Drawing for the job (mm, zero at the part's lowest x, y, z). A direction names the side the tool comes from. Round coordinates to 2 decimals unless told otherwise and drop trailing zeros. Order: outer loops, then holes, each group sorted by start corner. A loop starts at its lowest first (then second) coordinate and runs counter-clockwise, first axis right, second up. Notation, with made-up numbers: (-0.75, 88.25) -> (21.25, 88.25) arc R20 cw to (21.25, 97.25) -> close; hole circle Ø4 at (-38.75, 22.25). An arc over 180 degrees is marked (long way). Use CSV: the item, a comma, the result in double quotes.
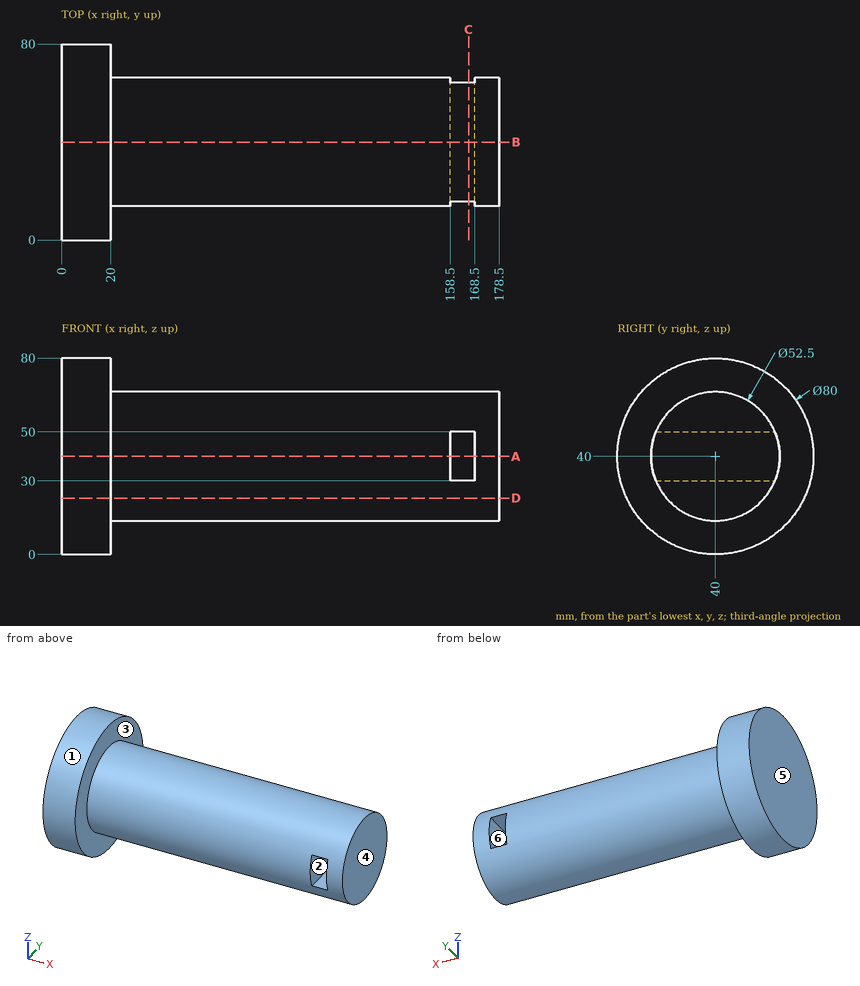
Q1. Cut at C-C (x = 166). Give the cut face in (y, z).
From the geometry:
outline,"(15.73, 30) arc R26.25 ccw to (64.27, 30) -> close; (15.73, 50) -> (64.27, 50) arc R26.25 ccw to start"
Q2. Which spindle directions (+Z, -Z, +X, -X, +Y, -Y) get a long thin tool onto all of the face, cutting with end or side? Do the marked faces 1, 2 and 3. Say none if no direction does.
From the geometry:
face 1,"+X, -X"
face 2,"+Y, -Y"
face 3,"+X"
Q3. Pin check, flat tips, straight feed: pin 1 (2 mm diameter, centred on x = 147.5, y = 59, fed in from -Z); pin 2 (1 mm diameter, centred on y = 59.5, z = 16.5, fed in from -X); pin 3 (8 mm diameter, centred on x = 161.5, y = 48.5, fed in from -Z); pin 4 (3 mm diameter, centred on x = 61, z = 62, fed in from +Y). Stop position of each tip, or through.
From the geometry:
pin 1,"stops at z = 20.89"
pin 2,"stops at x = 0"
pin 3,"stops at z = 14.14"
pin 4,"stops at y = 56.4"
Q4. Probe line 1 along X through (y, z) = (53.5, 44); line 2 along X through (y, z) = (59.5, 71); line 3 along Y through (x, z) = (133.5, 30). List the from-to ranges inside material, lowest first.
From the geometry:
line 1,"x = 0 to 158.5, 168.5 to 178.5"
line 2,"x = 0 to 20"
line 3,"y = 15.73 to 64.27"
Q5. Cut at B-B (y = 40). Give the cut face in (x, z), plus the area to 3 significant figures.
From the geometry:
outline,"(0, 0) -> (20, 0) -> (20, 13.75) -> (178.5, 13.75) -> (178.5, 66.25) -> (20, 66.25) -> (20, 80) -> (0, 80) -> close; hole (158.5, 30) -> (168.5, 30) -> (168.5, 50) -> (158.5, 50) -> close"
area,"9,720 mm²"
Q6. Cut at D-D (z = 23). Give the cut face in (x, y).
From the geometry:
outline,"(0, 3.79) -> (20, 3.79) -> (20, 20) -> (178.5, 20) -> (178.5, 60) -> (20, 60) -> (20, 76.21) -> (0, 76.21) -> close"
Q7. Mould opens along X. For the marked faces 4, 5 and 6 say: +X half, -X half, draft (parallel to the pull), parting line (faces both ways), or undercut.
From the geometry:
face 4,"+X half"
face 5,"-X half"
face 6,"undercut"
Q8. Cut at A-A (z = 40). Give the cut face in (x, y), plus the area to 3 significant figures.
From the geometry:
outline,"(0, 0) -> (20, 0) -> (20, 13.75) -> (158.5, 13.75) -> (158.5, 66.25) -> (20, 66.25) -> (20, 80) -> (0, 80) -> close; (168.5, 13.75) -> (178.5, 13.75) -> (178.5, 66.25) -> (168.5, 66.25) -> close"
area,"9,400 mm²"
